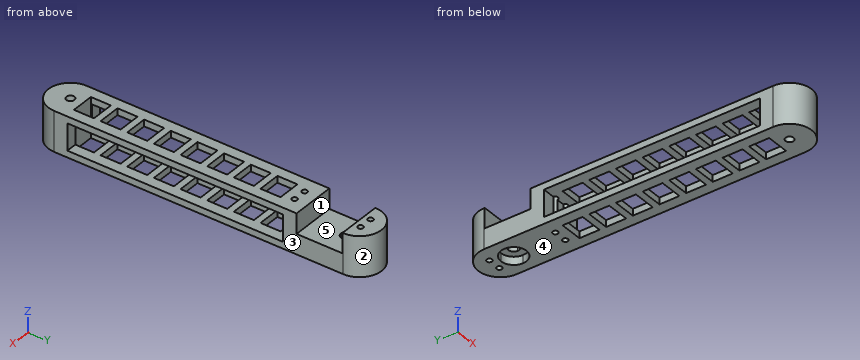
```python
from build123d import *

# Parameters (mm, degrees)
SKETCH1_R           = 2
SKETCH1_R_2         = 3
BOSS_EXTRUDE2_DEPTH = 30
CUT_EXTRUDE1_DEPTH  = 39
CUT_EXTRUDE2_DEPTH  = 6
SKETCH3_W           = 38.691948064
SKETCH3_H           = 34.5
CUT_EXTRUDE5_DEPTH  = 15
SKETCH4_W           = 17
SKETCH4_H           = 15
CUT_EXTRUDE6_DEPTH  = 33
SKETCH6_W           = 20
SKETCH6_H           = 162
CUT_EXTRUDE7_DEPTH  = 33


with BuildPart() as part:
    # Sketch1 → Boss-Extrude2 (new body)
    with BuildSketch(Plane.XY):
        with BuildLine():
            Line((-16.5, -41.885232007), (-16.5, 175.114767993))
            ThreePointArc((-16.5, 175.114767993), (0, 191.614767993), (16.5, 175.114767993))
            Line((16.5, 175.114767993), (16.5, -41.885232007))
            ThreePointArc((16.5, -41.885232007), (0, -58.385232007), (-16.5, -41.885232007))
        make_face()
        with Locations((5, 179.614767993)):
            Circle(SKETCH1_R, mode=Mode.SUBTRACT)
        with Locations((-5, 179.614767993)):
            Circle(SKETCH1_R, mode=Mode.SUBTRACT)
        with Locations((5, 130.114767993)):
            Circle(SKETCH1_R, mode=Mode.SUBTRACT)
        with Locations((-5, 130.114767993)):
            Circle(SKETCH1_R, mode=Mode.SUBTRACT)
        with Locations((0, -41.885232007)):
            Circle(SKETCH1_R_2, mode=Mode.SUBTRACT)
    extrude(amount=BOSS_EXTRUDE2_DEPTH)

    # Sketch1_4 → Cut-Extrude1 (cut)
    with BuildSketch(Plane.XY):
        with BuildLine():
            ThreePointArc((0, 169.114767993), (-4, 165.114767993), (0, 161.114767993))
            Line((0, 161.114767993), (0, 169.114767993))
        make_face()
        with BuildLine():
            Line((0, 169.114767993), (0, 161.114767993))
            ThreePointArc((0, 161.114767993), (2.828427125, 162.286340868), (4, 165.114767993))
            ThreePointArc((4, 165.114767993), (2.828427125, 167.943195117), (0, 169.114767993))
        make_face()
    extrude(amount=CUT_EXTRUDE1_DEPTH, mode=Mode.SUBTRACT)

    # Sketch1_5 → Cut-Extrude2 (cut)
    with BuildSketch(Plane.XY):
        with BuildLine():
            ThreePointArc((0, 174.614767993), (-9.5, 165.114767993), (0, 155.614767993))
            Line((0, 155.614767993), (0, 161.114767993))
            ThreePointArc((0, 161.114767993), (-4, 165.114767993), (0, 169.114767993))
            Line((0, 169.114767993), (0, 174.614767993))
        make_face()
        with BuildLine():
            Line((0, 161.114767993), (0, 155.614767993))
            ThreePointArc((0, 155.614767993), (6.717514421, 158.397253571), (9.5, 165.114767993))
            ThreePointArc((9.5, 165.114767993), (6.717514421, 171.832282414), (0, 174.614767993))
            Line((0, 174.614767993), (0, 169.114767993))
            ThreePointArc((0, 169.114767993), (2.828427125, 167.943195117), (4, 165.114767993))
            ThreePointArc((4, 165.114767993), (2.828427125, 162.286340868), (0, 161.114767993))
        make_face()
    extrude(amount=CUT_EXTRUDE2_DEPTH, mode=Mode.SUBTRACT)

    # Sketch3 → Cut-Extrude5 (cut)
    with BuildSketch(Plane.XY.offset(30)):
        with Locations((0.226361627, 157.364767993)):
            Rectangle(SKETCH3_W, SKETCH3_H)
    extrude(amount=-CUT_EXTRUDE5_DEPTH, mode=Mode.SUBTRACT)

    # Sketch4 → Cut-Extrude6 (cut)
    with BuildSketch(Plane.XY.offset(30)):
        with Locations((0, 114.614767993)):
            Rectangle(SKETCH4_W, SKETCH4_H)
        with Locations((0, 94.614767993)):
            Rectangle(SKETCH4_W, SKETCH4_H)
        with Locations((0, 74.614767993)):
            Rectangle(SKETCH4_W, SKETCH4_H)
        with Locations((0, 54.614767993)):
            Rectangle(SKETCH4_W, SKETCH4_H)
        with Locations((0, 34.614767993)):
            Rectangle(SKETCH4_W, SKETCH4_H)
        with Locations((0, 14.614767993)):
            Rectangle(SKETCH4_W, SKETCH4_H)
        with Locations((0, -5.385232007)):
            Rectangle(SKETCH4_W, SKETCH4_H)
        with Locations((0, -25.385232007)):
            Rectangle(SKETCH4_W, SKETCH4_H)
    extrude(amount=-CUT_EXTRUDE6_DEPTH, mode=Mode.SUBTRACT)

    # Sketch6 → Cut-Extrude7 (cut)
    with BuildSketch(Plane(origin=(16.5, 0, 0), x_dir=(0, 0, -1), z_dir=(1, 0, 0))):
        with Locations((-15, 49.114767993)):
            Rectangle(SKETCH6_W, SKETCH6_H)
    extrude(amount=-CUT_EXTRUDE7_DEPTH, mode=Mode.SUBTRACT)


solid = part.part
```
Here's how the part is built. I have some questions about the finished solid (model axes, mm). Face numbers are marked on the shaded views. A direction names the side the tool comes from. Coordinates: 2 decimals unless noted, no trailing zeros. Order: outer loops, then holes, each group sorted by start corner. A loop starts at its lowest first (then second) coordinate and runs counter-clockwise, first axis right, second up.
1) Imagine slicing it at B-B on z = 22. List the corners of the cut face in (x, y) for me.
2) We'd pull the mould along Y, two halves only. Please class the marked faces 1, 2 and 3: +Y half, -Y half, draft (parallel to the pull), parting line (faces both ways), or undercut.
3) Will these pins go through, and if not, where does the flat tip stop? pin 1 (1.8 mm diameter, centred on x = 0.5, z = 17, fed in from -Y); pin 2 (6 mm diameter, centred on x = 9, z = 26, fed in from +Y); pin 3 (1.5 mm diameter, centred on x = 3, z = 3, fed in from +Y); pin 4 (10.5 mm diameter, centred on x = 10.5, z = 16, fed in from -Y).
4) Imagine slicing it at C-C on x = -13.5. List the corners of the cut face in (y, z) for me, and give its area (3 significant figures).
5) Imagine slicing it at D-D on z = 2.75. State how many separate pieces and enclosed holes the cut face has, and give its area (3 significant figures).
6) Which directions (+Z, -Z, +X, -X, +Y, -Y) give clear straight access to the entire face, cutting with the end or side of a thin tool? Please do the marked faces 4 and 5.
7) I need wall thicknesses on line 1 (Y direction, x = 0.5, z = 12.75); line 2 (Y direction, x = 0, z = 15.5); line 3 (Z direction, x = -9, y = 101). Which ranges of each line are inside material? Lowest first, please.
8) Imagine slicing it at A-A on y = -20.5. List the corners of the cut face in (x, z) for me, and give its area (3 significant figures).
Response values:
1. outline: (-16.5, -41.89) arc R16.5 ccw to (16.5, -41.89) - (16.5, -31.89) - (8.5, -31.89) - (8.5, -32.89) - (-8.5, -32.89) - (-8.5, -31.89) - (-16.5, -31.89) - close; (-16.5, 130.11) - (-7, 130.11) arc R2 cw to (-3, 130.11) - (3, 130.11) arc R2 cw to (7, 130.11) - (16.5, 130.11) - (16.5, 140.11) - (-16.5, 140.11) - close; (-16.5, 174.61) - (16.5, 174.61) - (16.5, 175.11) arc R16.5 ccw to (-16.5, 175.11) - close; hole circle Ø4 at (-5, 179.61); hole circle Ø6 at (0, -41.89); hole circle Ø4 at (5, 179.61)
2. face 1: undercut
2. face 2: +Y half
2. face 3: draft
3. pin 1: stops at y = -58.39
3. pin 2: stops at y = 190.49
3. pin 3: stops at y = 191.46
3. pin 4: stops at y = -57.53
4. outline: (-51.37, 0) - (184.6, 0) - (184.6, 30) - (174.61, 30) - (174.61, 15) - (140.11, 15) - (140.11, 30) - (-51.37, 30) - close; hole (-31.89, 5) - (130.11, 5) - (130.11, 25) - (-31.89, 25) - close
4. area: 3,320 mm2
5. separate pieces: 1
5. enclosed holes: 14
5. area: 5,610 mm2
6. face 4: -Z, +X, -X, +Y, -Y
6. face 5: +Z, +X, -X
7. line 1: y = -58.38 to -44.84, -38.93 to -32.89, 130.11 to 161.15, 169.08 to 191.61
7. line 2: y = -58.39 to -44.89, -38.89 to -32.89, 130.11 to 140.11, 174.61 to 191.61
7. line 3: z = 0 to 5, 25 to 30
8. outline: (-16.5, 0) - (-8.5, 0) - (-8.5, 5) - (-16.5, 5) - close; (-16.5, 25) - (-8.5, 25) - (-8.5, 30) - (-16.5, 30) - close; (8.5, 0) - (16.5, 0) - (16.5, 5) - (8.5, 5) - close; (8.5, 25) - (16.5, 25) - (16.5, 30) - (8.5, 30) - close
8. area: 160 mm2
